Check sheet for the modelled part. Datum: model origin and axes. Units: mm. Face numbers are marked on the shaded views. A direction names the side the tool comes from. Give positions to 0.01 mm unless a question says otherwise; leave off trailing zeros. Order: outer loops, then holes, each group sorted by start corner. A loop starts at its lowest first (then second) coordinate and runs counter-clockwise, first axis right, second up. Notation, with made-up numbers: (-12, 45.5) - (32, 45.5) arc R17 ccw to (32, 74.5) - close; hole circle Ø2 at (-38.5, -25). An arc over 180 degrees is marked (long way). Answer in a Markdown table with one row per item.
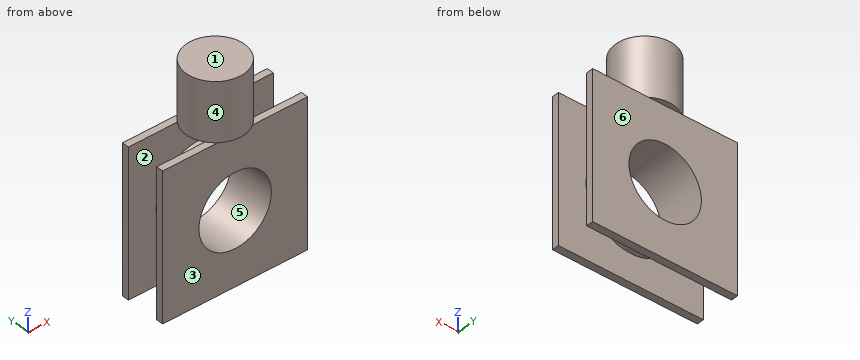
from build123d import *

# Parameters (mm, degrees)
SKETCH1_R                = 15.5
SKETCH1_R_2              = 12.5
BOSS_EXTRUDE1_DEPTH      = 15
SKETCH2_W                = 100
SKETCH2_H                = 2.435831537
SKETCH2_H_2              = 2.435831538
BOSS_EXTRUDE2_DEPTH      = 50
BOSS_EXTRUDE2_DEPTH_BACK = 50
SKETCH1_4_R              = 12.5
CUT_EXTRUDE1_DEPTH       = 20
SKETCH1_7_W              = 100
SKETCH1_7_H              = 100
SKETCH1_7_W_2            = 50
SKETCH1_7_H_2            = 50
CUT_EXTRUDE2_DEPTH       = 20
SKETCH4_R                = 10
BOSS_EXTRUDE3_DEPTH      = 20


with BuildPart() as part:
    # Sketch1 → Boss-Extrude1 (new body)
    with BuildSketch(Plane(origin=(0, 0, 0), x_dir=(1, 0, 0), z_dir=(0, 1, 0))):
        Circle(SKETCH1_R)
        Circle(SKETCH1_R_2, mode=Mode.SUBTRACT)
    extrude(amount=BOSS_EXTRUDE1_DEPTH)

    # Sketch2 → Boss-Extrude2 (add, two sides)
    with BuildSketch(Plane.XY) as boss_extrude2_sk:
        with Locations((0, 1.217915769)):
            Rectangle(SKETCH2_W, SKETCH2_H)
        with Locations((0, 15.01290923)):
            Rectangle(SKETCH2_W, SKETCH2_H_2)
    extrude(amount=BOSS_EXTRUDE2_DEPTH)
    extrude(boss_extrude2_sk.sketch, amount=-BOSS_EXTRUDE2_DEPTH_BACK)

    # Sketch1_4 → Cut-Extrude1 (cut)
    with BuildSketch(Plane(origin=(0, 0, 0), x_dir=(1, 0, 0), z_dir=(0, 1, 0))):
        Circle(SKETCH1_4_R)
    extrude(amount=CUT_EXTRUDE1_DEPTH, mode=Mode.SUBTRACT)

    # Sketch1_7 → Cut-Extrude2 (cut)
    with BuildSketch(Plane(origin=(0, 0, 0), x_dir=(1, 0, 0), z_dir=(0, 1, 0))):
        Rectangle(SKETCH1_7_W, SKETCH1_7_H)
        Rectangle(SKETCH1_7_W_2, SKETCH1_7_H_2, mode=Mode.SUBTRACT)
    extrude(amount=CUT_EXTRUDE2_DEPTH, mode=Mode.SUBTRACT)

    # Sketch4 → Boss-Extrude3 (add)
    with BuildSketch(Plane.XY.offset(25)):
        with Locations((0, 8)):
            Circle(SKETCH4_R)
    extrude(amount=BOSS_EXTRUDE3_DEPTH)


solid = part.part
(1) Thickness scan on L1, parallel to Z at x = 0, y = 5.25; L2, parallel to Y at x = 8.5, z = -13.5 (3 decimals); L3, parallel to Z at x = -5.5, y = 15. Record the ranges inside material, lowest first.
Geometry says:
| item | result |
|---|---|
| L1 | -15.5 to -12.5, 12.5 to 15.5, 25 to 45 |
| L2 | 0 to 2.436, 13.795 to 16.231 |
| L3 | -25 to -11.22, 11.22 to 45 |
(2) Cross-section at B-B, the plane x = 0. Record the cut outline in (y, z) (3 decimals), then the cut area to 3 significant figures.
Geometry says:
| item | result |
|---|---|
| outline | (-2, 25) - (0, 25) - (0, 12.5) - (16.231, 12.5) - (16.231, 25) - (18, 25) - (18, 45) - (-2, 45) - close; (0, -25) - (2.436, -25) - (2.436, -15.5) - (13.795, -15.5) - (13.795, -25) - (16.231, -25) - (16.231, -12.5) - (0, -12.5) - close; hole (2.436, 15.5) - (13.795, 15.5) - (13.795, 25) - (2.436, 25) - close |
| area | 590 mm² |
(3) Access from +Z, -Z, +X, -X, +Y, -Y to the whole of each face (thin tool, end or side, straight path). Record for the marked faces 1, 2 and 3.
Geometry says:
| item | result |
|---|---|
| face 1 | +Z, +X, -X, +Y, -Y |
| face 2 | none |
| face 3 | -Z, +X, -X, -Y |
(4) Cross-section at D-D, the plane x = 17.5. Record the cut outline in (y, z) (3 decimals).
Geometry says:
| item | result |
|---|---|
| outline | (0, -25) - (2.436, -25) - (2.436, 25) - (0, 25) - close; (13.795, -25) - (16.231, -25) - (16.231, 25) - (13.795, 25) - close |
(5) Cross-section at C-C, the plane y = 8. Record the cut outline in (x, z).
Geometry says:
| item | result |
|---|---|
| outline | circle Ø31 at (0, 0); (-10, 25) - (10, 25) - (10, 45) - (-10, 45) - close; hole circle Ø25 at (0, 0) |
(6) Gauge pin test, flat ends, axial feed: P1, Ø2.5, axis at x = 19, y = 2, coming from the +Z side; P2, Ø3, axis at x = 12, y = 8, coming from the +Z side; P3, Ø3.5, axis at x = -1, y = 10, coming from the -Z side. Record the tip position at first contact, or that the pin passes through.
Geometry says:
| item | result |
|---|---|
| P1 | z = 25 |
| P2 | z = 11.4 |
| P3 | z = -15.5 |
(7) Cross-section at A-A, the plane z = 0. Record the cut outline in (x, y) (3 decimals), then the cut area to 3 significant figures.
Geometry says:
| item | result |
|---|---|
| outline | (-25, 0) - (-12.5, 0) - (-12.5, 16.231) - (-25, 16.231) - (-25, 13.795) - (-15.5, 13.795) - (-15.5, 2.436) - (-25, 2.436) - close; (12.5, 0) - (25, 0) - (25, 2.436) - (15.5, 2.436) - (15.5, 13.795) - (25, 13.795) - (25, 16.231) - (12.5, 16.231) - close |
| area | 190 mm² |
(8) Mould release check, pull along X, two halves, no side actions. Record for the marked faces 4, 5 and 6: pulls with the +X half, pulls with the -X half, needs draft (parallel to the pull), parting line crosses it, or undercut.
Geometry says:
| item | result |
|---|---|
| face 4 | parting line crosses it |
| face 5 | undercut |
| face 6 | needs draft |
